Design review of the part built by this model. Coordinates are the model's own, in mm. A direction names the side the tool comes from. Round coordinates to 2 decimals unless told otherwise and drop trailing zeros. Loops run counter-clockwise (first coordinate to the right, second up) from the corner with the lowest first, then second, coordinate; pieces in that order, holes last. Notation, with made-up numbers: (24.25, 73) -> (71.25, 73) arc R21 ccw to (71.25, 78) -> close; hole circle Ø7 at (35.5, 46). An arc over 180 degrees is marked (long way). Write each question's results on one line, items separated by ' | '. Start each with the question number.
Solid Edge part; units mm, degrees
sketch "Sketch1" plane through (0, 0, 0) normal (0, 0, 1) x (1, 0, 0)
  line L0 (-46, -29) -> (46, -29)
  line L1 (46, -29) -> (46, 29)
  line L2 (46, 29) -> (-46, 29)
  line L3 (-46, 29) -> (-46, -29)
  dimension "D1" = 46
  dimension "D2" = 46
extrude "Ajout_matière_1" add sketch "Sketch1" along normal mid plane 5
sketch "Sketch2" plane through (46, 0, 0) normal (1, 0, 0) x (0, 1, 0)
  circle A0 centre (0, -5.5) radius 6
extrude "Cutout1" cut sketch "Sketch2" against normal through all
hole "Perçage_1" at (-43.5, 26.5, 2.5) direction (0, 0, -1) diameter 3.1 end up to next
hole "Hole1" at (43.5, 26.5, 2.5) direction (0, 0, -1) diameter 3.1 end up to next
hole "Hole2" at (43.5, -26.5, 2.5) direction (0, 0, -1) diameter 3.1 end up to next
hole "Hole3" at (-43.5, -26.5, 2.5) direction (0, 0, -1) diameter 3.1 end up to next
hole "Hole4" at (-39, 24.5, 2.5) direction (0, 0, -1) diameter 2.5 end up to next
hole "Hole5" at (19, 24.5, 2.5) direction (0, 0, -1) diameter 2.5 end up to next
hole "Hole6" at (19, -24.5, 2.5) direction (0, 0, -1) diameter 2.5 end up to next
hole "Hole7" at (-39, -24.5, 2.5) direction (0, 0, -1) diameter 2.5 end up to next
sketch "Sketch3" plane through (0, 0, 2.5) normal (0, 0, 1) x (0, 1, 0)
  circle A0 centre (-24.5, 39) radius 3
  circle A1 centre (-24.5, 39) radius 1.25
  circle A2 centre (24.5, 39) radius 1.25
  circle A3 centre (24.5, 39) radius 3
  circle A4 centre (24.5, -19) radius 1.25
  circle A5 centre (24.5, -19) radius 3
  circle A6 centre (-24.5, -19) radius 1.25
  circle A7 centre (-24.5, -19) radius 3
extrude "Protrusion1" add sketch "Sketch3" along normal blind 2
properties material "Plastique ABS, performance moyenne"
1) The part is to be moulded in two halves that separate along Y. For faces 1 (the face through (1, 29, 0)), 2 (the face through (-36.026, -24.891, 3.486)), 3 (the face through (19, 23, 4.5)), say which applies: +Y half, -Y half, draft (parallel to the pull), parting line (faces both ways), or undercut.
2) Take a section at A-A (z = -1.5). State how many separate pieces and enclosed holes the cut face has, plus the area to 3 significant figures.
3) Insertion check: pin 1 (4 mm diameter, centred on x = -43.5, y = -26.5, fed in from +Z); pin 2 (2 mm diameter, centred on x = 19, y = -24.5, fed in from +Z); pin 3 (5 mm diameter, centred on x = 43.5, y = 26.5, fed in from +Z). Each pin has a flat end and moves straight along its axis. Give the tip position at first contact, or say it passes through.
4) Take a section at B-B (x = -43.5). Write out the cut boundary in (y, z).
5) For faces 4 (the face through (-39, -26, 4.5)), 5 (the face through (16.07, -25.15, 3.49)), list the 3-axis set-ups (+Z, -Z, +X, -X, +Y, -Y) from which the entire face can be reached by the end or side of a thin tool; tool diameter is ignored.
6) Take a section at D-D (y = 12). Write out the cut boundary in (x, z).
7) Take a section at C-C (x = 19). Write out the cut boundary in (y, z).
8) To check wall thickness, follow line 1 (X direction, y = 26.5, z = -0.1); line 2 (X direction, y = 24.5, z = 1.3); line 3 (X direction, y = -24.5, z = 3.5). State the ranges of each line that lie inside material, in increasing order. Write a range as from..to.
Geometry check:
1) face 1: +Y half | face 2: undercut | face 3: draft
2) separate pieces: 2 | enclosed holes: 8 | area: 4,460 mm^2
3) pin 1: stops at z = 4.5 | pin 2: passes through | pin 3: stops at z = 2.5
4) outline: (-29, -2.5) -> (-28.05, -2.5) -> (-28.05, 2.5) -> (-29, 2.5) -> close; (-24.95, -2.5) -> (-5.2, -2.5) arc R6 cw to (5.2, -2.5) -> (24.95, -2.5) -> (24.95, 2.5) -> (-24.95, 2.5) -> close; (28.05, -2.5) -> (29, -2.5) -> (29, 2.5) -> (28.05, 2.5) -> close
5) face 4: +Z, +X, -X, +Y, -Y | face 5: +Z
6) outline: (-46, -2.5) -> (46, -2.5) -> (46, 2.5) -> (-46, 2.5) -> close
7) outline: (-29, -2.5) -> (-25.75, -2.5) -> (-25.75, 4.5) -> (-27.5, 4.5) -> (-27.5, 2.5) -> (-29, 2.5) -> close; (-23.25, -2.5) -> (-5.2, -2.5) arc R6 cw to (5.2, -2.5) -> (23.25, -2.5) -> (23.25, 4.5) -> (21.5, 4.5) -> (21.5, 2.5) -> (-21.5, 2.5) -> (-21.5, 4.5) -> (-23.25, 4.5) -> close; (25.75, -2.5) -> (29, -2.5) -> (29, 2.5) -> (27.5, 2.5) -> (27.5, 4.5) -> (25.75, 4.5) -> close
8) line 1: x = -46..-45.05, -41.95..41.95, 45.05..46 | line 2: x = -46..-40.25, -37.75..17.75, 20.25..46 | line 3: x = -42..-40.25, -37.75..-36, 16..17.75, 20.25..22
